from build123d import *

# Parameters (mm, degrees)
F0_R     = 9
F0_R_2   = 7.5
F0_R_3   = 5
F1_DEPTH = 16
F2_DEPTH = 14
F3_DEPTH = 4
F4_R     = 2
F5_DEPTH = 12.5


with BuildPart() as f1:
    # F0 (on Top) → F1 (new body)
    with BuildSketch(Plane.XY):
        Circle(F0_R)
        Circle(F0_R_2, mode=Mode.SUBTRACT)
        Circle(F0_R_2)
        Circle(F0_R_3, mode=Mode.SUBTRACT)
        Circle(F0_R_3)
    extrude(amount=F1_DEPTH)

    # F0 (on Top) → F2 (cut)
    with BuildSketch(Plane.XY):
        Circle(F0_R_3)
    extrude(amount=F2_DEPTH, mode=Mode.SUBTRACT)

    # F0 (on Top) → F3 (cut)
    with BuildSketch(Plane.XY):
        Circle(F0_R_2)
        Circle(F0_R_3, mode=Mode.SUBTRACT)
    extrude(amount=F3_DEPTH, mode=Mode.SUBTRACT)

    # F4 (on Front) → F5 (cut, symmetric)
    with BuildSketch(Plane.XZ):
        with Locations((0, 8)):
            Circle(F4_R)
    extrude(amount=F5_DEPTH, both=True, mode=Mode.SUBTRACT)


solid = f1.part
Input: part model. Units: mm. Frame: model coordinates. A direction names the side the tool comes from. Coordinates: 2 decimals unless noted, no trailing zeros. Order: outer loops, then holes, each group sorted by start corner. A loop starts at its lowest first (then second) coordinate and runs counter-clockwise, first axis right, second up. Notation, with made-up numbers: M -19,-40 L 12,-40 A12 cw 12,-18 Z; hole C 61,6 d11. An arc over 180 degrees is marked long. Answer in a Markdown table with one row per item.
(1) Section query A-A, the plane x = 0. Output: boundary loops of the cut face in (y, z).
Numbers:
| item | result |
|---|---|
| outline | M -9,0 L -7.5,0 L -7.5,4 L -5,4 L -5,6 L -9,6 Z; M -9,10 L -5,10 L -5,14 L 5,14 L 5,10 L 9,10 L 9,16 L -9,16 Z; M 5,4 L 7.5,4 L 7.5,0 L 9,0 L 9,6 L 5,6 Z |
(2) Section query B-B, the plane y = 0. Output: boundary loops of the cut face in (x, z).
Numbers:
| item | result |
|---|---|
| outline | M -9,0 L -7.5,0 L -7.5,4 L -5,4 L -5,14 L 5,14 L 5,4 L 7.5,4 L 7.5,0 L 9,0 L 9,16 L -9,16 Z |
(3) Section query D-D, the plane z = 8. Output: boundary loops of the cut face in (x, y), plus the area to 3 significant figures.
Numbers:
| item | result |
|---|---|
| outline | M -2,-8.77 L -2,-4.58 A5 cw -2,4.58 L -2,8.77 A9 ccw Z; M 2,-8.77 A9 ccw 2,8.77 L 2,4.58 A5 cw 2,-4.58 Z |
| area | 143 mm^2 |
(4) Contact query for flat-ended pins moving along their axis: pin 1 Ø4 at (x, z) = (5, 14) entering from -Y; pin 2 Ø4 at (x, z) = (-5.5, 3) entering from +Y; pin 3 Ø7.5 at (x, y) = (2, 0) entering from -Z; pin 4 Ø3 at (x, z) = (0, 8) entering from +Y. Output: stop coordinate, or through.
Numbers:
| item | result |
|---|---|
| pin 1 | stops at y = -8.49 |
| pin 2 | stops at y = 8.29 |
| pin 3 | stops at z = 4 |
| pin 4 | passes through |
(5) Access query for faces 1 (the flat face through (0, 0, 16)), 2 (the cylindrical face through (-7.493, 0.33, 1.972)). Directions: +Z, -Z, +X, -X, +Y, -Y. A direction counts if a zero-diameter tool reaches every point of the face in a straight line with its end or side. Return the directions, or none.
Numbers:
| item | result |
|---|---|
| face 1 | +Z, +X, -X, +Y, -Y |
| face 2 | -Z |
(6) Section query C-C, the plane y = 7.25. Output: boundary loops of the cut face in (x, z), plus the area to 3 significant figures.
Numbers:
| item | result |
|---|---|
| outline | M -5.33,0 L -1.92,0 L -1.92,4 L 1.92,4 L 1.92,0 L 5.33,0 L 5.33,16 L -5.33,16 Z; hole C 0,8 d4 |
| area | 143 mm^2 |
(7) Draft query along Y for faces 3 (the cylindrical face through (8.584, 2.703, 7.888)), 4 (the cylindrical face through (-2, 7, 8)), 5 (the flat face through (2, -5, 4)), 6 (the cylindrical face through (4.619, -1.915, 8.93)). Return one class per face: pulls with the +Y half, pulls with the -Y half, needs draft (parallel to the pull), parting line crosses it, or undercut.
Numbers:
| item | result |
|---|---|
| face 3 | parting line crosses it |
| face 4 | needs draft |
| face 5 | undercut |
| face 6 | undercut |
(8) Material intervals for line 1 (Y direction, x = 0, z = 1.8); line 2 (Z direction, x = 3.75, y = 1.75); line 3 (Y direction, x = 3.75, z = 8.5), sorted ascending. Write a range as [from, to].
Numbers:
| item | result |
|---|---|
| line 1 | y = [-9, -7.5], [7.5, 9] |
| line 2 | z = [14, 16] |
| line 3 | y = [-8.18, -3.31], [3.31, 8.18] |
